```python
from build123d import *
from build123d.topology import SkipClean

# Parameters (mm, degrees)
SALIENTE_EXTRUIR4_DEPTH    = 6
CROQUIS10_R                = 1.03
SALIENTE_EXTRUIR5_DEPTH    = 3
CROQUIS10_3_R              = 1.03
CORTAR_EXTRUIR7_DEPTH      = 6
CORTAR_EXTRUIR8_REACH      = 20
CORTAR_EXTRUIR8_END_RADIUS = 12
CROQUIS11_R                = 2
CORTAR_EXTRUIR11_START     = 9
CROQUIS11_3_R              = 2.5
CORTAR_EXTRUIR11_DEPTH     = 10.000000167
CORTAR_EXTRUIR9_START      = 4.6
CORTAR_EXTRUIR9_DEPTH      = 2.6
CORTAR_EXTRUIR12_REACH     = 20
CORTAR_EXTRUIR10_START     = -3
CORTAR_EXTRUIR10_DEPTH     = 3
CORTAR_EXTRUIR13_START     = -9
CROQUIS11_5_R              = 2.5
CORTAR_EXTRUIR13_DEPTH     = 10.000000167
CORTAR_EXTRUIR14_START     = -2
CORTAR_EXTRUIR14_DEPTH     = 2.6
CORTAR_EXTRUIR15_START     = -3
CORTAR_EXTRUIR15_DEPTH     = 3
SALIENTE_EXTRUIR6_DEPTH    = 1
CORTAR_EXTRUIR17_DEPTH     = 2


with BuildPart() as part:
    # Croquis1 → Saliente-Extruir4 (new body)
    with BuildSketch(Plane(origin=(0, 0, 0), x_dir=(1, 0, 0), z_dir=(0, 1, 0))):
        with BuildLine():
            Line((0, -12), (0, 0))
            Line((0, 0), (-12, 0))
            ThreePointArc((-12, 0), (-8.485281374, -8.485281374), (0, -12))
        make_face()
        with BuildLine():
            Line((-12, 0), (0, 0))
            Line((0, 0), (0, 12))
            ThreePointArc((0, 12), (-8.485281374, 8.485281374), (-12, 0))
        make_face()
        with BuildLine():
            Line((0, 12), (0, 0))
            Line((0, 0), (12, 0))
            ThreePointArc((12, 0), (8.485281374, 8.485281374), (0, 12))
        make_face()
        with BuildLine():
            Line((12, 0), (0, 0))
            Line((0, 0), (0, -12))
            ThreePointArc((0, -12), (8.485281374, -8.485281374), (12, 0))
        make_face()
    extrude(amount=SALIENTE_EXTRUIR4_DEPTH)

    # Croquis10 → Saliente-Extruir5 (add)
    with BuildSketch(Plane(origin=(0, 0, 0), x_dir=(1, 0, 0), z_dir=(0, 1, 0))):
        Circle(CROQUIS10_R)
    extrude(amount=SALIENTE_EXTRUIR5_DEPTH)

    # Croquis10<3> → Cortar-Extruir7 (cut)
    with BuildSketch(Plane(origin=(0, 0, 0), x_dir=(1, 0, 0), z_dir=(0, 1, 0))):
        with Locations(Location((0, 0, 0), (0, 0, 270))):
            Circle(CROQUIS10_3_R)
    extrude(amount=CORTAR_EXTRUIR7_DEPTH, mode=Mode.SUBTRACT)

    # Cortar-Extruir8: up to this cylinder (the profile starts inside it)
    cortar_extruir8_end = Plane(origin=(0, 3, 0), z_dir=(0, -1, 0)) * Cylinder(CORTAR_EXTRUIR8_END_RADIUS, 65, mode=Mode.PRIVATE)
    # Croquis11 → Cortar-Extruir8 (cut, up to the surface)
    with BuildSketch(Plane(origin=(0, 0, 0), x_dir=(0.7071067811865477, 0, -0.7071067811865475), z_dir=(0.7071067811865475, 0, 0.7071067811865477)), mode=Mode.PRIVATE) as cortar_extruir8_sk1:
        with Locations(Location((0, 3, 0), (0, 0, 180))):
            Circle(CROQUIS11_R)
    cortar_extruir8_tool1 = extrude(cortar_extruir8_sk1.sketch, amount=CORTAR_EXTRUIR8_REACH, mode=Mode.PRIVATE) & cortar_extruir8_end
    add(cortar_extruir8_tool1.solids().sort_by_distance((0, 3, 0))[0], mode=Mode.SUBTRACT)

    # Croquis11<3> → Cortar-Extruir11 (cut, through all)
    with BuildSketch(Plane(origin=(0, 0, 0), x_dir=(0.7071067811865477, 0, -0.7071067811865475), z_dir=(0.7071067811865475, 0, 0.7071067811865477)).offset(CORTAR_EXTRUIR11_START)):
        with Locations(Location((0, 3, 0), (0, 0, 180))):
            Circle(CROQUIS11_3_R)
    extrude(amount=CORTAR_EXTRUIR11_DEPTH, mode=Mode.SUBTRACT)

    # Croquis14 → Cortar-Extruir9 (cut)
    with BuildSketch(Plane(origin=(0, 0, 0), x_dir=(0.7071067811865477, 0, -0.7071067811865475), z_dir=(0.7071067811865475, 0, 0.7071067811865477)).offset(CORTAR_EXTRUIR9_START)):
        Polygon((1.327905619, 5.3), (-1.327905619, 5.3), (-2.655811238, 3), (-1.327905619, 0.7), (1.327905619, 0.7), (2.655811238, 3), align=None)
    extrude(amount=-CORTAR_EXTRUIR9_DEPTH, mode=Mode.SUBTRACT)

    # Croquis11<4> → Cortar-Extruir12 (cut, up to next)
    with BuildSketch(Plane(origin=(0, 0, 0), x_dir=(0.7071067811865477, 0, -0.7071067811865475), z_dir=(0.7071067811865475, 0, 0.7071067811865477)), mode=Mode.PRIVATE) as cortar_extruir12_sk1:
        with BuildLine():
            ThreePointArc((2, 3), (1.414213562, 4.414213562), (0, 5))
            Line((0, 5), (0, 1))
            ThreePointArc((0, 1), (1.414213562, 1.585786438), (2, 3))
        make_face()
    cortar_extruir12_tool1 = extrude(cortar_extruir12_sk1.sketch, amount=-CORTAR_EXTRUIR12_REACH, mode=Mode.PRIVATE) & part.part
    # Croquis11<4> → Cortar-Extruir12 (cut, up to next)
    with BuildSketch(Plane(origin=(0, 0, 0), x_dir=(0.7071067811865477, 0, -0.7071067811865475), z_dir=(0.7071067811865475, 0, 0.7071067811865477)), mode=Mode.PRIVATE) as cortar_extruir12_sk2:
        with BuildLine():
            Line((0, 1), (0, 5))
            ThreePointArc((0, 5), (-2, 3), (0, 1))
        make_face()
    cortar_extruir12_tool2 = extrude(cortar_extruir12_sk2.sketch, amount=-CORTAR_EXTRUIR12_REACH, mode=Mode.PRIVATE) & part.part
    # Croquis11<4> → Cortar-Extruir12 (cut, up to next)
    with BuildSketch(Plane(origin=(0, 0, 0), x_dir=(0.7071067811865477, 0, -0.7071067811865475), z_dir=(0.7071067811865475, 0, 0.7071067811865477)), mode=Mode.PRIVATE) as cortar_extruir12_sk3:
        with BuildLine():
            ThreePointArc((2, 3), (1.414213562, 4.414213562), (0, 5))
            Line((0, 5), (0, 1))
            ThreePointArc((0, 1), (1.414213562, 1.585786438), (2, 3))
        make_face()
    cortar_extruir12_tool3 = extrude(cortar_extruir12_sk3.sketch, amount=-CORTAR_EXTRUIR12_REACH, mode=Mode.PRIVATE) & part.part
    # Croquis11<4> → Cortar-Extruir12 (cut, up to next)
    with BuildSketch(Plane(origin=(0, 0, 0), x_dir=(0.7071067811865477, 0, -0.7071067811865475), z_dir=(0.7071067811865475, 0, 0.7071067811865477)), mode=Mode.PRIVATE) as cortar_extruir12_sk4:
        with BuildLine():
            Line((0, 1), (0, 5))
            ThreePointArc((0, 5), (-2, 3), (0, 1))
        make_face()
    cortar_extruir12_tool4 = extrude(cortar_extruir12_sk4.sketch, amount=-CORTAR_EXTRUIR12_REACH, mode=Mode.PRIVATE) & part.part
    add(cortar_extruir12_tool1.solids().sort_by_distance((0.600211, 3, -0.600211))[0], mode=Mode.SUBTRACT)
    add(cortar_extruir12_tool2.solids().sort_by_distance((-0.600211, 3, 0.600211))[0], mode=Mode.SUBTRACT)
    add(cortar_extruir12_tool3.solids().sort_by_distance((0.600211, 3, -0.600211))[0], mode=Mode.SUBTRACT)
    add(cortar_extruir12_tool4.solids().sort_by_distance((-0.600211, 3, 0.600211))[0], mode=Mode.SUBTRACT)

    # Croquis16 → Cortar-Extruir10 (cut)
    with SkipClean():  # the faces are left unmerged after this step: merging them gives an invalid solid
        with BuildSketch(Plane(origin=(0, 6, 0), x_dir=(1, 0, 0), z_dir=(0, 1, 0)).offset(CORTAR_EXTRUIR10_START)):
            Polygon((-0.463728574, -3.292155699), (1.374749057, -5.13063333), (5.13063333, -1.374749057), (3.292155699, 0.463728574), align=None)
        extrude(amount=CORTAR_EXTRUIR10_DEPTH, mode=Mode.SUBTRACT)

    # Croquis11<5> → Cortar-Extruir13 (cut, through all)
    with BuildSketch(Plane(origin=(0, 0, 0), x_dir=(0.7071067811865477, 0, -0.7071067811865475), z_dir=(0.7071067811865475, 0, 0.7071067811865477)).offset(CORTAR_EXTRUIR13_START)):
        with Locations(Location((0, 3, 0), (0, 0, 180))):
            Circle(CROQUIS11_5_R)
    extrude(amount=-CORTAR_EXTRUIR13_DEPTH, mode=Mode.SUBTRACT)

    # Croquis14<2> → Cortar-Extruir14 (cut)
    with BuildSketch(Plane(origin=(0, 0, 0), x_dir=(0.7071067811865477, 0, -0.7071067811865475), z_dir=(0.7071067811865475, 0, 0.7071067811865477)).offset(CORTAR_EXTRUIR14_START)):
        Polygon((1.327905619, 5.3), (-1.327905619, 5.3), (-2.655811238, 3), (-1.327905619, 0.7), (1.327905619, 0.7), (2.655811238, 3), align=None)
    extrude(amount=-CORTAR_EXTRUIR14_DEPTH, mode=Mode.SUBTRACT)

    # Croquis18 → Cortar-Extruir15 (cut)
    with BuildSketch(Plane(origin=(0, 6, 0), x_dir=(1, 0, 0), z_dir=(0, 1, 0)).offset(CORTAR_EXTRUIR15_START)):
        Polygon((0.463728574, 3.292155699), (-3.292155699, -0.463728574), (-5.13063333, 1.374749057), (-1.374749057, 5.13063333), align=None)
    extrude(amount=CORTAR_EXTRUIR15_DEPTH, mode=Mode.SUBTRACT)

    # Croquis1<11> → Saliente-Extruir6 (add)
    with BuildSketch(Plane(origin=(0, 0, 0), x_dir=(1, 0, 0), z_dir=(0, 1, 0))):
        with BuildLine():
            Line((0, 19), (0, 12))
            ThreePointArc((0, 12), (8.485281374, 8.485281374), (12, 0))
            Line((12, 0), (19, 0))
            ThreePointArc((19, 0), (13.435028843, 13.435028843), (0, 19))
        make_face()
        with BuildLine():
            Line((0, 22), (0, 19))
            ThreePointArc((0, 19), (13.435028843, 13.435028843), (19, 0))
            Line((19, 0), (22, 0))
            ThreePointArc((22, 0), (15.556349186, 15.556349186), (0, 22))
        make_face()
        with BuildLine():
            Line((0, -22), (0, -19))
            ThreePointArc((0, -19), (-13.435028843, -13.435028843), (-19, 0))
            Line((-19, 0), (-22, 0))
            ThreePointArc((-22, 0), (-15.556349186, -15.556349186), (0, -22))
        make_face()
        with BuildLine():
            Line((0, -19), (0, -12))
            ThreePointArc((0, -12), (-8.485281374, -8.485281374), (-12, 0))
            Line((-12, 0), (-19, 0))
            ThreePointArc((-19, 0), (-13.435028843, -13.435028843), (0, -19))
        make_face()
        with BuildLine():
            Line((22, 0), (19, 0))
            ThreePointArc((19, 0), (13.435028843, -13.435028843), (0, -19))
            Line((0, -19), (0, -22))
            ThreePointArc((0, -22), (15.556349186, -15.556349186), (22, 0))
        make_face()
        with BuildLine():
            ThreePointArc((-19, 0), (-13.435028843, 13.435028843), (0, 19))
            Line((0, 19), (0, 22))
            ThreePointArc((0, 22), (-15.556349186, 15.556349186), (-22, 0))
            Line((-22, 0), (-19, 0))
        make_face()
        with BuildLine():
            Line((19, 0), (12, 0))
            ThreePointArc((12, 0), (8.485281374, -8.485281374), (0, -12))
            Line((0, -12), (0, -19))
            ThreePointArc((0, -19), (13.435028843, -13.435028843), (19, 0))
        make_face()
        with BuildLine():
            ThreePointArc((-12, 0), (-8.485281374, 8.485281374), (0, 12))
            Line((0, 12), (0, 19))
            ThreePointArc((0, 19), (-13.435028843, 13.435028843), (-19, 0))
            Line((-19, 0), (-12, 0))
        make_face()
    extrude(amount=SALIENTE_EXTRUIR6_DEPTH)

    # Croquis20 → Cortar-Extruir17 (cut)
    with SkipClean():  # the faces are left unmerged after this step: merging them gives an invalid solid
        with BuildSketch(Plane.XZ):
            with BuildLine():
                Line((5.085233412, 18.306840283), (3.211726365, 11.562214916))
                ThreePointArc((3.211726365, 11.562214916), (7.391916343, 9.453019242), (10.446754065, 5.90468708))
                Line((10.446754065, 5.90468708), (16.540693936, 9.349087877))
                ThreePointArc((16.540693936, 9.349087877), (11.703867543, 14.967280466), (5.085233412, 18.306840283))
            make_face()
            with BuildLine():
                Line((18.306840283, -5.085233412), (11.562214916, -3.211726365))
                ThreePointArc((11.562214916, -3.211726365), (9.453019242, -7.391916343), (5.90468708, -10.446754065))
                Line((5.90468708, -10.446754065), (9.349087877, -16.540693936))
                ThreePointArc((9.349087877, -16.540693936), (14.967280466, -11.703867543), (18.306840283, -5.085233412))
            make_face()
            with BuildLine():
                Line((-5.085233412, -18.306840283), (-3.211726365, -11.562214916))
                ThreePointArc((-3.211726365, -11.562214916), (-7.391916343, -9.453019242), (-10.446754065, -5.90468708))
                Line((-10.446754065, -5.90468708), (-16.540693936, -9.349087877))
                ThreePointArc((-16.540693936, -9.349087877), (-11.703867543, -14.967280466), (-5.085233412, -18.306840283))
            make_face()
            with BuildLine():
                Line((-18.306840283, 5.085233412), (-11.562214916, 3.211726365))
                ThreePointArc((-11.562214916, 3.211726365), (-9.453019242, 7.391916343), (-5.90468708, 10.446754065))
                Line((-5.90468708, 10.446754065), (-9.349087877, 16.540693936))
                ThreePointArc((-9.349087877, 16.540693936), (-14.967280466, 11.703867543), (-18.306840283, 5.085233412))
            make_face()
        extrude(amount=-CORTAR_EXTRUIR17_DEPTH, mode=Mode.SUBTRACT)


solid = part.part
```
CAD build for the part. Positions are in the model's coordinates, mm. A direction names the side the tool comes from. Round coordinates to 2 decimals unless told otherwise and drop trailing zeros. Order: outer loops, then holes, each group sorted by start corner. A loop starts at its lowest first (then second) coordinate and runs counter-clockwise, first axis right, second up.
Item 1: Tool access for faces 4 (the face through (1.1, 3.37, -1.68)), 5 (the face through (-14.98, 0.49, 4.16)), 6 (the face through (2, 0.7, 2)): list every direction of +Z, -Z, +X, -X, +Y, -Y with a clear straight run to the whole face (end or side of a thin tool).
Item 2: Pin check, flat tips, straight feed: pin 1 (1 mm diameter, centred on y = 2.5, z = -9.5, fed in from -X); pin 2 (2 mm diameter, centred on y = 4, z = -11, fed in from +X); pin 3 (4 mm diameter, centred on x = 17, z = 15.5, fed in from +Y). Stop position of each tip, or through.
Item 3: Probe line 1 along X through (y, z) = (1.05, 0); line 2 along Z through (x, y) = (0, 5.25). List the from-to ranges inside material, lowest first.
Item 4: Saw through at D-D on x = -15.5. Write the cut outline in (y, z), then the cut area to 3 significant figures.
Item 5: Saw through at B-B on z = 11. Write the cut outline in (x, y), then the cut area to 3 significant figures.
Item 6: Mould opens along X. For faces 1 (the face through (3.748, 1.834, 0.944)), 2 (the face through (2, 6, 0)), 3 (the face through (4.224, 4.479, 0.468)) say: pulls with the +X half, pulls with the -X half, needs draft (parallel to the pull), parting line crosses it, or undercut.
Item 7: Saw through at A-A on x = 16. Write the cut outline in (y, z), then the cut area to 3 significant figures.
Reported:
1. face 4: none
1. face 5: +Y, -Y
1. face 6: +Y
2. pin 1: stops at x = -6.56
2. pin 2: stops at x = 6.63
2. pin 3: stops at y = 1
3. line 1: x = -12 to -1.03, 1.03 to 12
3. line 2: z = -12 to -3.76, -2.83 to -1.03, 1.03 to 2.83, 3.76 to 12
4. outline: (0, -15.61) - (1, -15.61) - (1, -10.99) - (0, -10.99) - close; (0, -8.76) - (1, -8.76) - (1, 4.31) - (0, 4.31) - close; (0, 10.99) - (1, 10.99) - (1, 15.61) - (0, 15.61) - close
4. area: 22.3 mm2
5. outline: (-19.05, 0) - (-15.49, 0) - (-15.49, 1) - (-19.05, 1) - close; (-6.22, 0) - (4.8, 0) - (4.8, 6) - (-4.8, 6) - (-4.8, 1) - (-6.22, 1) - close; (15.49, 0) - (19.05, 0) - (19.05, 1) - (15.49, 1) - close
5. area: 66.1 mm2
6. face 1: undercut
6. face 2: needs draft
6. face 3: undercut
7. outline: (0, -15.1) - (1, -15.1) - (1, -10.25) - (0, -10.25) - close; (0, -4.44) - (1, -4.44) - (1, 9.04) - (0, 9.04) - close; (0, 10.25) - (1, 10.25) - (1, 15.1) - (0, 15.1) - close
7. area: 23.2 mm2
